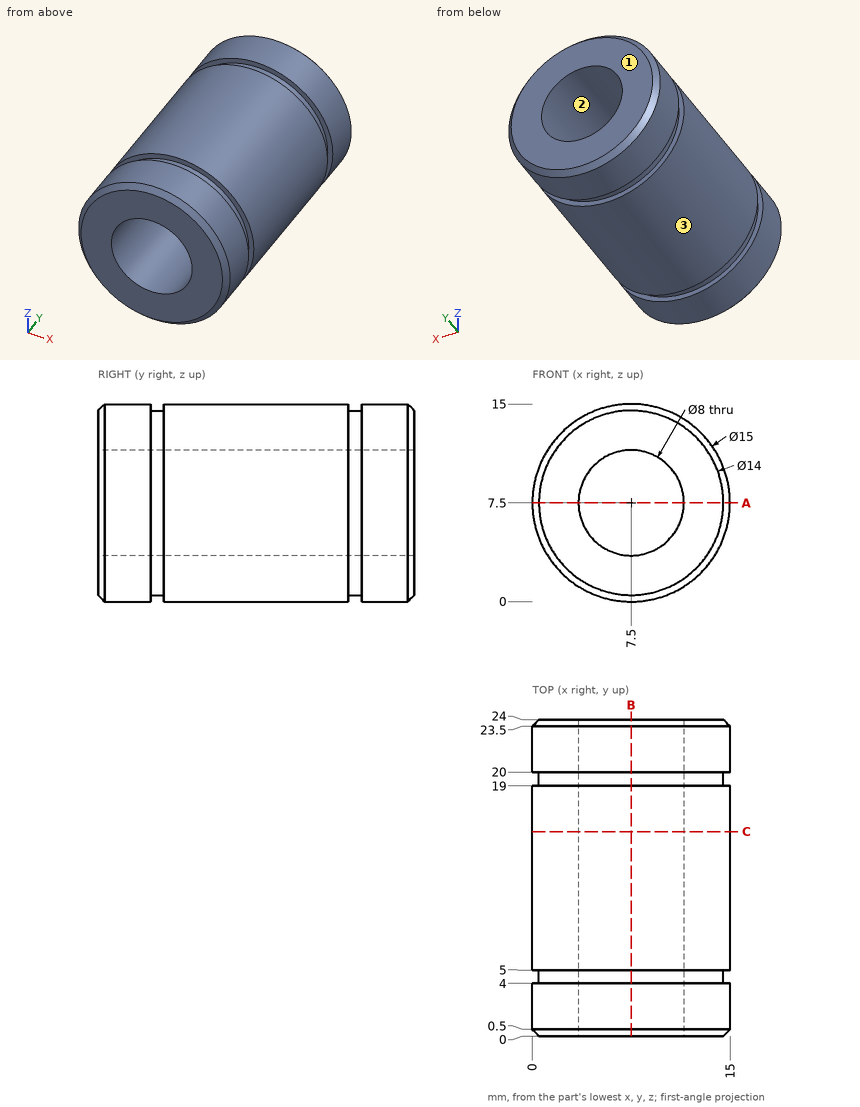
Geometry check sheet. Reference: drawing and pictorial views, mm from the part's lowest x, y, z. Coordinates: 2 decimals unless noted, no trailing zeros. Write each loop counter-clockwise with the first axis right and the second up, starting at its lowest first coordinate (ties: lowest second). Pieces come first, ordered by that corner, then holes. Notation, with made-up numbers: M 21,-8 L 29,-8 A26 ccw 29,18 Z; hole C 75.5,0 d2. An arc over 180 degrees is marked long. Write item = value, one per line. Start each with the question number.
1. Go/stop test with flat-tipped pins: pin 1 (1 mm diameter, centred on y = 9.5, z = 8.5, fed in from -X); pin 2 (4.5 mm diameter, centred on x = 8.5, z = 7, fed in from +Y); pin 3 (2 mm diameter, centred on x = 11, y = 13, fed in from -Z). Record where each tip stops, or that it passes through.
2. Sectioned sample at C-C (y = 15.5). Record the cut outline in (x, z), then the cut area to 3 significant figures.
3. Sectioned sample at A-A (z = 7.5). Record the cut outline in (x, y), then the cut area to 4 significant figures.
4. Thickness scan on probe 1 along Z at (x, y) = (7.5, 18.5); probe 2 along Y at (x, z) = (14.25, 5); probe 3 along Y at (x, z) = (14.5, 8.5). Record the ranges inside material, lowest first.
5. Sectioned sample at B-B (x = 7.5). Record the cut outline in (y, z).
6. Mould release check, pull along X, two halves, no side actions. Record for the marked faces 1, 2 and 3: pulls with the +X half, pulls with the -X half, needs draft (parallel to the pull), parting line crosses it, or undercut.
The answers:
q1.pin_1 = 0.02
q1.pin_2 = through
q1.pin_3 = 0.43
q2.outline = C 7.5,7.5 d15; hole C 7.5,7.5 d8
q2.area = 126 mm²
q3.outline = M 0,0.5 L 0.5,0 L 3.5,0 L 3.5,24 L 0.5,24 L 0,23.5 L 0,20 L 0.5,20 L 0.5,19 L 0,19 L 0,5 L 0.5,5 L 0.5,4 L 0,4 Z; M 11.5,0 L 14.5,0 L 15,0.5 L 15,4 L 14.5,4 L 14.5,5 L 15,5 L 15,19 L 14.5,19 L 14.5,20 L 15,20 L 15,23.5 L 14.5,24 L 11.5,24 Z
q3.area = 165.5 mm²
q4.probe_1 = 0 to 3.5, 11.5 to 15
q4.probe_2 = 0.2 to 4, 5 to 19, 20 to 23.8
q4.probe_3 = 0.07 to 4, 5 to 19, 20 to 23.93
q5.outline = M 0,0.5 L 0.5,0 L 4,0 L 4,0.5 L 5,0.5 L 5,0 L 19,0 L 19,0.5 L 20,0.5 L 20,0 L 23.5,0 L 24,0.5 L 24,3.5 L 0,3.5 Z; M 0,11.5 L 24,11.5 L 24,14.5 L 23.5,15 L 20,15 L 20,14.5 L 19,14.5 L 19,15 L 5,15 L 5,14.5 L 4,14.5 L 4,15 L 0.5,15 L 0,14.5 Z
q6.face_1 = needs draft
q6.face_2 = undercut
q6.face_3 = parting line crosses it
